Geometry: final body of the model. Coordinates: model frame, mm. Face numbers are marked on the shaded views. A direction names the side the tool comes from. Coordinates: 2 decimals unless noted, no trailing zeros. Order: outer loops, then holes, each group sorted by start corner. A loop starts at its lowest first (then second) coordinate and runs counter-clockwise, first axis right, second up. Notation, with made-up numbers: M -34,84 L 7,84 A31 cw 7,112 Z; hole C 73.25,63 d3. An arc over 180 degrees is marked long. Use CSV: the item, a comma, the result in double quotes. Start each with the question number.
1. Set-up query: the marked faces 1, 2 and 3. Return all of +Z, -Z, +X, -X, +Y, -Y with unobstructed straight access to the full face (end or side cutting, diameter ignored); none if empty.
2. Section query A-A on z = 65.5. Return the cut outline in (x, y) (3 decimals), and give its area (3 significant figures).
3. Section query C-C on z = 10. Return the cut outline in (x, y), and give its area (3 significant figures).
4. Section query D-D on y = 112. Return the cut outline in (x, z) (3 decimals), and give its area (3 significant figures).
5. Section query B-B on y = 93. Return the cut outline in (x, z) (3 decimals), and give its area (3 significant figures).
6. First-contact query: P1, Ø4.5, axis at x = 21.5, y = 17.5, coming from the -Z side; P2, Ø5, axis at x = 22, y = 82.5, coming from the +Z side; P3, Ø6, axis at x = 34.5, z = 25.5, coming from the -Y side; P4, Ø5, axis at y = 58, z = 61, coming from the -X side (3 decimals). Flat tips, straight axial feed; report the tip coordinate or a pass-through.
7. Pull-direction query (X, two-part tool) for the marked faces 4, 5, 6 and 7; classes: pulls with the +X half, pulls with the -X half, needs draft (parallel to the pull), parting line crosses it, or undercut.
8. Material intervals for line 1 (X direction, y = 46, z = 15); line 2 (Z direction, x = 14.5, y = 7.5); line 3 (X direction, y = 0.75, z = 27.5) (3 decimals), sorted ascending.
from build123d import *

# Parameters (mm, degrees)
SKETCH1_W           = 43.57
SKETCH1_H           = 63.5
BOSS_EXTRUDE1_DEPTH = 55
CUT_EXTRUDE2_DEPTH  = 95.634004988
SKETCH4_W           = 43.57
SKETCH4_H           = 55
SKETCH4_W_2         = 6
SKETCH4_H_2         = 15
BOSS_EXTRUDE2_DEPTH = 9
SKETCH5_R           = 1
CUT_EXTRUDE3_DEPTH  = 1
BOSS_EXTRUDE3_START = -26.785
BOSS_EXTRUDE3_DEPTH = 10
SKETCH7_R           = 2
CUT_EXTRUDE4_DEPTH  = 2
SKETCH13_W          = 9
SKETCH13_H          = 8
BOSS_EXTRUDE6_DEPTH = 10
FILLET12_R          = 3
FILLET2_R           = 1
BOSS_EXTRUDE4_DEPTH = 10
BOSS_EXTRUDE5_DEPTH = 7.5
CUT_EXTRUDE11_DEPTH = 174.835946297
LPATTERN1_COUNT     = 5
LPATTERN1_PITCH     = 12
FILLET9_R           = 1
FILLET11_R          = 11
SKETCH14_R          = 2
CUT_EXTRUDE12_DEPTH = 156.361674811
SKETCH15_W          = 15
SKETCH15_H          = 33
CUT_EXTRUDE13_DEPTH = 33
SKETCH16_W          = 15
SKETCH16_H          = 25
CUT_EXTRUDE14_DEPTH = 26
SKETCH18_R          = 1.016
CUT_EXTRUDE15_DEPTH = 8
SKETCH19_W          = 15
SKETCH19_H          = 5
CUT_EXTRUDE16_DEPTH = 25
SKETCH20_W          = 38.57
SKETCH20_H          = 51
CUT_EXTRUDE17_DEPTH = 33
SKETCH21_W          = 4
SKETCH21_H          = 13
CUT_EXTRUDE18_DEPTH = 27
SKETCH22_W          = 10
SKETCH22_H          = 40.521468164
BOSS_EXTRUDE7_DEPTH = 8
FILLET13_R          = 2
FILLET14_R          = 2


with BuildPart() as part:
    # Sketch1 → Boss-Extrude1 (new body)
    with BuildSketch(Plane.XY):
        with Locations((21.785, 31.75)):
            Rectangle(SKETCH1_W, SKETCH1_H)
    extrude(amount=BOSS_EXTRUDE1_DEPTH)

    # Sketch3 → Cut-Extrude2 (cut, through all)
    with BuildSketch(Plane(origin=(43.57, 0, 0), x_dir=(0, 0, -1), z_dir=(1, 0, 0))):
        with BuildLine():
            Line((-29.5, 0), (-29.5, 1.5))
            ThreePointArc((-29.5, 1.5), (-29.060660172, 2.560660172), (-28, 3))
            Line((-28, 3), (-27, 3))
            ThreePointArc((-27, 3), (-25.939339828, 2.560660172), (-25.5, 1.5))
            Line((-25.5, 1.5), (-25.5, 0))
            Line((-25.5, 0), (-22.5, 0))
            Line((-22.5, 0), (-22.5, 3.5))
            ThreePointArc((-22.5, 3.5), (-22.939339828, 4.560660172), (-24, 5))
            Line((-24, 5), (-31, 5))
            ThreePointArc((-31, 5), (-32.060660172, 4.560660172), (-32.5, 3.5))
            Line((-32.5, 3.5), (-32.5, 0))
            Line((-32.5, 0), (-29.5, 0))
        make_face()
    extrude(amount=-CUT_EXTRUDE2_DEPTH, mode=Mode.SUBTRACT)


with BuildPart() as cut_extrude2_piece_1:
    # of the separate pieces the step leaves, piece 1, a body of its own (cut_extrude2_pieces)
    add(part.part.solids().sort_by_distance((0, 0, 0))[0])



with BuildPart() as cut_extrude2_piece_2:
    # of the separate pieces the step leaves, piece 2, a body of its own (cut_extrude2_pieces)
    add(part.part.solids().sort_by_distance((43.57, 0, 25.5))[0])


with BuildPart() as cut_extrude2_piece_1_1:
    add(cut_extrude2_piece_1.part)

    add(cut_extrude2_piece_2.part)  # Boss-Extrude2 merges Cut-Extrude2 piece 2
    # Sketch4 → Boss-Extrude2 (add)
    with BuildSketch(Plane.XZ):
        with Locations((21.785, 27.5)):
            Rectangle(SKETCH4_W, SKETCH4_H)
        with Locations((10.785, 27.5)):
            Rectangle(SKETCH4_W_2, SKETCH4_H_2, mode=Mode.SUBTRACT)
        with Locations((32.785, 27.5)):
            Rectangle(SKETCH4_W_2, SKETCH4_H_2, mode=Mode.SUBTRACT)
    extrude(amount=-BOSS_EXTRUDE2_DEPTH)

    # Sketch5 → Cut-Extrude3 (cut)
    with BuildSketch(Plane(origin=(0, 0, 0), x_dir=(-1, 0, 0), z_dir=(0, -1, 0))):
        with Locations(Location((-21.785, -27.5, 0), (0, 0, 90))):
            Circle(SKETCH5_R)
    extrude(amount=-CUT_EXTRUDE3_DEPTH, mode=Mode.SUBTRACT)

    # Sketch6 → Boss-Extrude3 (add)
    with BuildSketch(Plane.ZY.offset(BOSS_EXTRUDE3_START)):
        with BuildLine():
            Line((55, 48.5), (75, 48.5))
            ThreePointArc((75, 48.5), (80, 53.5), (75, 58.5))
            Line((75, 58.5), (55, 58.5))
            ThreePointArc((55, 58.5), (50, 53.5), (55, 48.5))
        make_face()
    boss_extrude3 = extrude(amount=BOSS_EXTRUDE3_DEPTH)

    # Mirror1: Boss-Extrude3 across plane
    add(boss_extrude3.mirror(Plane(origin=(0, 0, 27.5), x_dir=(1, 0, 0), z_dir=(0, 0, -1))))

    # Sketch7 → Cut-Extrude4 (cut, symmetric)
    # profile 1 of 3: a face of its own
    with BuildSketch(Plane.ZY.offset(-21.785)):
        with BuildLine():
            ThreePointArc((75, 58.5), (71.464466094, 57.035533906), (70, 53.5))
            ThreePointArc((70, 53.5), (71.464466094, 49.964466094), (75, 48.5))
            ThreePointArc((75, 48.5), (78.535533906, 49.964466094), (80, 53.5))
            ThreePointArc((80, 53.5), (78.535533906, 57.035533906), (75, 58.5))
        make_face()
        with Locations(Location((75, 53.5, 0), (0, 0, 270))):
            Circle(SKETCH7_R, mode=Mode.SUBTRACT)
    # profile 2 of 3: a face of its own
    with BuildSketch(Plane.ZY.offset(-21.785)):
        with BuildLine():
            Line((70, 58.5), (70, 53.5))
            ThreePointArc((70, 53.5), (71.464466094, 57.035533906), (75, 58.5))
            Line((75, 58.5), (70, 58.5))
        make_face()
    # profile 3 of 3: a face of its own
    with BuildSketch(Plane.ZY.offset(-21.785)):
        with BuildLine():
            ThreePointArc((75, 48.5), (71.464466094, 49.964466094), (70, 53.5))
            Line((70, 53.5), (70, 48.5))
            Line((70, 48.5), (75, 48.5))
        make_face()
    extrude(amount=CUT_EXTRUDE4_DEPTH, both=True, mode=Mode.SUBTRACT)

    # Sketch13 → Boss-Extrude6 (add)
    with BuildSketch(Plane(origin=(26.785, 0, 0), x_dir=(0, 0, -1), z_dir=(1, 0, 0))):
        with Locations((-65.5, 62.5)):
            Rectangle(SKETCH13_W, SKETCH13_H)
    extrude(amount=-BOSS_EXTRUDE6_DEPTH)

    # Fillet12
    fillet12_edges = [cut_extrude2_piece_1_1.edges().sort_by_distance(p)[0] for p in [
        (21.785, 66.5, 61),
        (21.785, 66.5, 70),
        (21.785, 58.5, 61),
    ]]
    fillet(fillet12_edges, radius=FILLET12_R)

    # Fillet2
    fillet2_edges = [cut_extrude2_piece_1_1.edges().sort_by_distance(p)[0] for p in [
        (16.785, 48.5, 65),
        (16.785, 53.5, 80),
        (16.785, 58.5, 72.5),
        (26.785, 48.5, 65),
        (26.785, 53.5, 80),
        (26.785, 58.5, 72.5),
    ]]
    fillet(fillet2_edges, radius=FILLET2_R)

    # Sketch10 → Boss-Extrude4 (add)
    with BuildSketch(Plane.ZY.offset(-16.785)):
        with BuildLine():
            Line((-25, 53.5), (-25, 78.5))
            Line((-25, 78.5), (-17.5, 78.5))
            Line((-17.5, 78.5), (-17.5, 58.5))
            Line((-17.5, 58.5), (-20, 58.5))
            ThreePointArc((-20, 58.5), (-23.535533906, 57.035533906), (-25, 53.5))
        make_face()
    extrude(amount=-BOSS_EXTRUDE4_DEPTH)

    # Sketch11 → Boss-Extrude5 (add)
    with BuildSketch(Plane(origin=(0, 0, -25), x_dir=(-1, 0, 0), z_dir=(0, 0, -1))):
        Polygon((-21.785, 63.5), (8.215, 78.5), (8.215, 128.5), (-51.785, 128.5), (-51.785, 78.5), align=None)
    extrude(amount=-BOSS_EXTRUDE5_DEPTH)

    # Sketch12 → Cut-Extrude11 (cut, through all)
    with BuildSketch(Plane(origin=(0, 0, -25), x_dir=(-1, 0, 0), z_dir=(0, 0, -1))):
        Polygon((-51.785, 128.5), (-45.785, 122.5), (-39.785, 128.5), align=None)
    cut_extrude11 = extrude(amount=-CUT_EXTRUDE11_DEPTH, mode=Mode.SUBTRACT)

    # LPattern1: Cut-Extrude11 ×5
    with Locations(*[(-i * LPATTERN1_PITCH, 0, 0) for i in range(1, LPATTERN1_COUNT)]):
        add(cut_extrude11, mode=Mode.SUBTRACT)

    # Fillet9
    fillet9_edges = [cut_extrude2_piece_1_1.edges().sort_by_distance(p)[0] for p in [
        (-8.215, 128.5, -21.25),
        (51.785, 128.5, -21.25),
    ]]
    fillet(fillet9_edges, radius=FILLET9_R)

    # Fillet11
    fillet11_edges = [cut_extrude2_piece_1_1.edges().sort_by_distance(p)[0] for p in [
        (-8.215, 78.5, -21.25),
        (51.785, 78.5, -21.25),
    ]]
    fillet(fillet11_edges, radius=FILLET11_R)

    # Sketch14 → Cut-Extrude12 (cut, through all)
    with BuildSketch(Plane.ZY.offset(-16.785)):
        with Locations(Location((65.5, 63, 0), (0, 0, 270))):
            Circle(SKETCH14_R)
    extrude(amount=-CUT_EXTRUDE12_DEPTH, mode=Mode.SUBTRACT)

    # Sketch15 → Cut-Extrude13 (cut)
    with BuildSketch(Plane(origin=(0, 63.5, 0), x_dir=(1, 0, 0), z_dir=(0, 1, 0))):
        with Locations((21.785, -27.5)):
            Rectangle(SKETCH15_W, SKETCH15_H)
    extrude(amount=-CUT_EXTRUDE13_DEPTH, mode=Mode.SUBTRACT)

    # Sketch16 → Cut-Extrude14 (cut)
    with BuildSketch(Plane(origin=(0, 30.5, 0), x_dir=(1, 0, 0), z_dir=(0, 1, 0))):
        with Locations((21.785, -27.5)):
            Rectangle(SKETCH16_W, SKETCH16_H)
    extrude(amount=-CUT_EXTRUDE14_DEPTH, mode=Mode.SUBTRACT)

    # Sketch18 → Cut-Extrude15 (cut)
    with BuildSketch(Plane(origin=(0, 30.5, 0), x_dir=(1, 0, 0), z_dir=(0, 1, 0))):
        with Locations(Location((21.785, -13.6, 0), (0, 0, 270))):
            Circle(SKETCH18_R)
        with Locations(Location((21.785, -41.4, 0), (0, 0, 270))):
            Circle(SKETCH18_R)
    extrude(amount=-CUT_EXTRUDE15_DEPTH, mode=Mode.SUBTRACT)

    # Sketch19 → Cut-Extrude16 (cut)
    with BuildSketch(Plane(origin=(0, 4.5, 0), x_dir=(1, 0, 0), z_dir=(0, 1, 0))):
        with Locations((21.785, -17.5)):
            Rectangle(SKETCH19_W, SKETCH19_H)
    extrude(amount=-CUT_EXTRUDE16_DEPTH, mode=Mode.SUBTRACT)

    # Sketch20 → Cut-Extrude17 (cut)
    with BuildSketch(Plane(origin=(0, 63.5, 0), x_dir=(1, 0, 0), z_dir=(0, 1, 0))):
        with Locations((21.785, -27.5)):
            Rectangle(SKETCH20_W, SKETCH20_H)
    extrude(amount=-CUT_EXTRUDE17_DEPTH, mode=Mode.SUBTRACT)

    # Sketch21 → Cut-Extrude18 (cut)
    with BuildSketch(Plane.XY.offset(70)):
        with Locations((21.785, 52)):
            Rectangle(SKETCH21_W, SKETCH21_H)
    extrude(amount=-CUT_EXTRUDE18_DEPTH, mode=Mode.SUBTRACT)

    # Sketch22 → Boss-Extrude7 (add)
    with BuildSketch(Plane.XY.offset(-17.5)):
        with Locations((21.785, 78.760734082)):
            Rectangle(SKETCH22_W, SKETCH22_H)
    extrude(amount=BOSS_EXTRUDE7_DEPTH)

    # Fillet13
    fillet13_edges = [cut_extrude2_piece_1_1.edges().sort_by_distance(p)[0] for p in [
        (16.785, 99.021468164, -13.5),
        (26.785, 99.021468164, -13.5),
    ]]
    fillet(fillet13_edges, radius=FILLET13_R)

    # Fillet14
    fillet14_edges = [cut_extrude2_piece_1_1.edges().sort_by_distance(p)[0] for p in [
        (26.785, 77.760734082, -9.5),
        (21.785, 99.021468164, -9.5),
        (16.785, 77.760734082, -9.5),
        (17.370786438, 98.435681727, -9.5),
        (26.199213562, 98.435681727, -9.5),
    ]]
    fillet(fillet14_edges, radius=FILLET14_R)


solid = cut_extrude2_piece_1_1.part
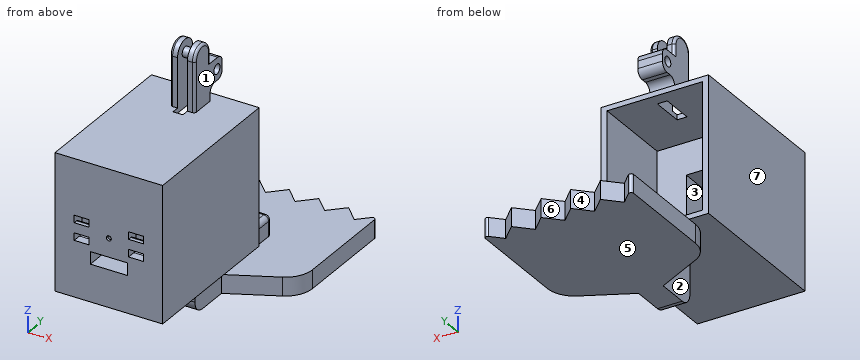
Results list:
1,face 1,"+Z, +X, +Y, -Y"
1,face 2,"-X, -Y"
1,face 3,"+Y"
2,outline,"M 16.785,49.5 A1 ccw 17.785,48.5 L 19.785,48.5 L 19.785,58.5 L 23.785,58.5 L 23.785,48.5 L 25.785,48.5 A1 ccw 26.785,49.5 L 26.785,61 L 16.785,61 Z; M 16.785,65 L 26.785,65 L 26.785,66.5 L 16.785,66.5 Z"
2,area,"99.6 mm²"
3,outline,"M 0,0 L 43.57,0 L 43.57,63.5 L 41.07,63.5 L 41.07,30.5 L 2.5,30.5 L 2.5,63.5 L 0,63.5 Z"
3,area,"1,490 mm²"
4,outline,"M -8.215,-25 L 51.785,-25 L 51.785,-17.5 L -8.215,-17.5 Z"
4,area,"450 mm²"
5,outline,"M -8.215,-25 L 51.785,-25 L 51.785,-17.5 L 26.785,-17.5 L 26.785,-11.5 A2 ccw 24.785,-9.5 L 18.785,-9.5 A2 ccw 16.785,-11.5 L 16.785,-17.5 L -8.215,-17.5 Z"
5,area,"528 mm²"
6,P1,"stops at z = 0"
6,P2,"stops at z = -9.5"
6,P3,"stops at y = 0"
6,P4,"stops at x = 16.785"
7,face 4,"undercut"
7,face 5,"needs draft"
7,face 6,"undercut"
7,face 7,"pulls with the -X half"
8,line 1,"x = 0 to 2.5, 41.07 to 43.57"
8,line 2,"z = 0 to 15, 40 to 55"
8,line 3,"x = 0 to 20.785, 22.785 to 43.57"
